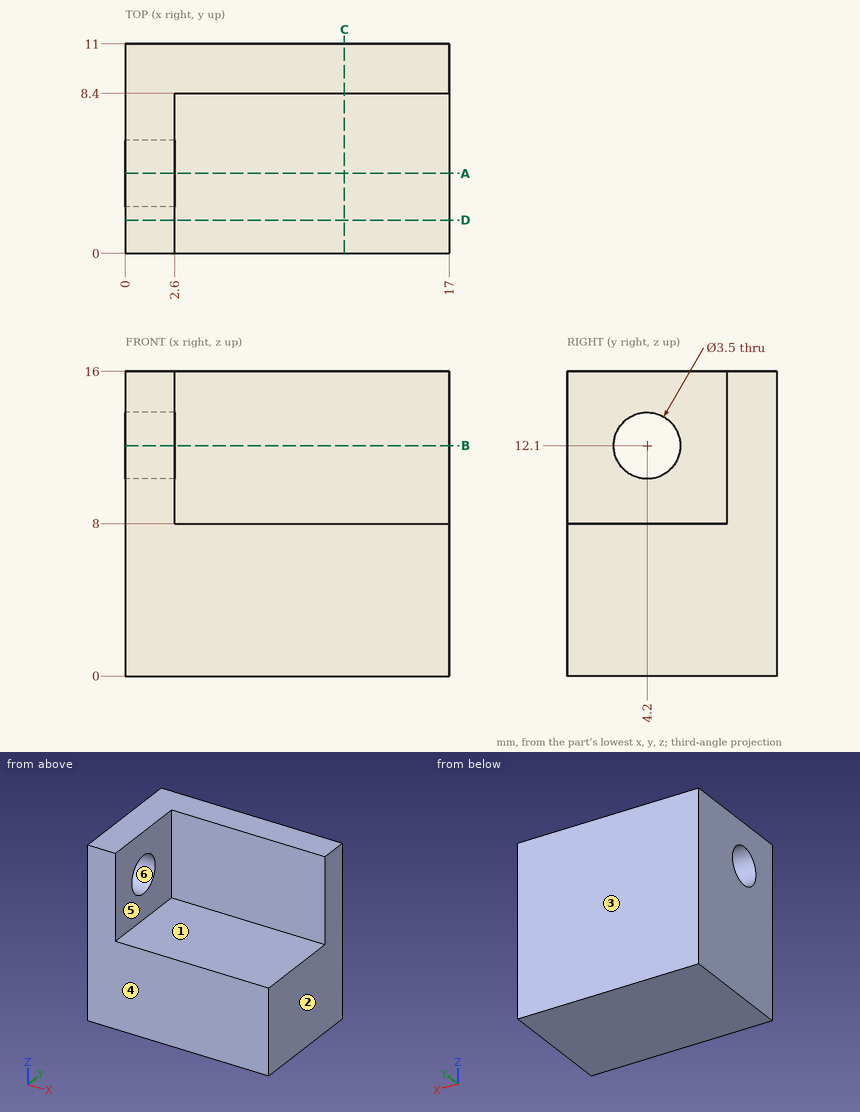
Check sheet for the drawn part. Datum: minimum x, y, z corner. Units: mm. A direction names the side the tool comes from. Give positions to 0.01 mm unless a question says otherwise; leave off trailing zeros. Order: outer loops, then holes, each group sorted by start corner. A loop starts at its lowest first (then second) coordinate and runs counter-clockwise, first axis right, second up. Notation, with made-up numbers: (62, 84.25) -> (87, 84.25) arc R15 ccw to (87, 98.25) -> close; hole circle Ø2 at (-28.5, -6.75). An arc over 180 degrees is marked (long way). Use a Markdown table: item, result.
1) Mould release check, pull along Y, two halves, no side actions. Record for the marked faces 3, 4, 5 and 6: pulls with the +Y half, pulls with the -Y half, needs draft (parallel to the pull), parting line crosses it, or undercut.
Results:
| item | result |
|---|---|
| face 3 | pulls with the +Y half |
| face 4 | pulls with the -Y half |
| face 5 | needs draft |
| face 6 | undercut |
2) Tool access check on the marked faces 1 and 2. Record the directions out of +Z, -Z, +X, -X, +Y, -Y that give a thin tool (end or side, any length) a straight path to the whole face; none if there is none.
Results:
| item | result |
|---|---|
| face 1 | +Z, +X, -Y |
| face 2 | +Z, -Z, +X, +Y, -Y |
3) Section check B-B, the plane z = 12.1. Record the boundary of the cut face in (x, y).
Results:
| item | result |
|---|---|
| outline | (0, 0) -> (2.6, 0) -> (2.6, 2.45) -> (0, 2.45) -> close; (0, 5.95) -> (2.6, 5.95) -> (2.6, 8.4) -> (17, 8.4) -> (17, 11) -> (0, 11) -> close |
4) Depth check by flat-ended pin: pin 1 Ø4 at (x, y) = (10, 3.5) entering from +Z; pin 2 Ø4 at (y, z) = (4.2, 12.1) entering from +X; pin 3 Ø2.5 at (x, z) = (6.5, 13) entering from -Y. Enter the tip coordinate at first touch or a pass-through.
Results:
| item | result |
|---|---|
| pin 1 | z = 8 |
| pin 2 | x = 2.6 |
| pin 3 | y = 8.4 |
5) Section check A-A, the plane y = 4.2. Record the boundary of the cut face in (x, z).
Results:
| item | result |
|---|---|
| outline | (0, 0) -> (17, 0) -> (17, 8) -> (2.6, 8) -> (2.6, 10.35) -> (0, 10.35) -> close; (0, 13.85) -> (2.6, 13.85) -> (2.6, 16) -> (0, 16) -> close |
6) Section check D-D, the plane y = 1.75. Record the boundary of the cut face in (x, z), then the cut area to 3 significant figures.
Results:
| item | result |
|---|---|
| outline | (0, 0) -> (17, 0) -> (17, 8) -> (2.6, 8) -> (2.6, 16) -> (0, 16) -> close |
| area | 157 mm² |
7) Material ranges on probe 1 along Z at (x, y) = (1.85, 4.2); probe 2 along Z at (x, y) = (8.5, 3.25); probe 3 along X at (y, z) = (3.5, 10), recorded low to high.
Results:
| item | result |
|---|---|
| probe 1 | 0 to 10.35, 13.85 to 16 |
| probe 2 | 0 to 8 |
| probe 3 | 0 to 2.6 |
8) Section check C-C, the plane x = 11.5. Record the boundary of the cut face in (y, z), then the cut area to 3 significant figures.
Results:
| item | result |
|---|---|
| outline | (0, 0) -> (11, 0) -> (11, 16) -> (8.4, 16) -> (8.4, 8) -> (0, 8) -> close |
| area | 109 mm² |
